The model under review builds one solid part; all positions refer to its coordinate system, in mm. Coordinates: 2 decimals unless noted, no trailing zeros. Loops run counter-clockwise (first coordinate to the right, second up) from the corner with the lowest first, then second, coordinate; pieces in that order, holes last. Notation, with made-up numbers: M 55,-17.5 L 69,-17.5 A4 ccw 69,-11.5 Z; hole C 86,-9.75 d11. An arc over 180 degrees is marked long. Use one line per item in the form item = value.
```python
from build123d import *

# Parameters (mm, degrees)
SKETCH1_R           = 1.524
SKETCH1_W           = 3.175
SKETCH1_H           = 3.175
BOSS_EXTRUDE1_DEPTH = 3.175


with BuildPart() as part:
    # Sketch1 → Boss-Extrude1 (new body)
    with BuildSketch(Plane(origin=(0, 0, 0), x_dir=(0, 0, -1), z_dir=(1, 0, 0))):
        with BuildLine():
            Line((-6.35, -285.75), (6.35, -285.75))
            Line((6.35, -285.75), (10.159096581, -0.135486743))
            ThreePointArc((10.159096581, -0.135486743), (0, 10.16), (-10.159096581, -0.135486743))
            Line((-10.159096581, -0.135486743), (-6.35, -285.75))
        make_face()
        Circle(SKETCH1_R, mode=Mode.SUBTRACT)
        with Locations((0, -10.668)):
            Circle(SKETCH1_R, mode=Mode.SUBTRACT)
        with Locations((0, -5.334)):
            Rectangle(SKETCH1_W, SKETCH1_H, mode=Mode.SUBTRACT)
    extrude(amount=BOSS_EXTRUDE1_DEPTH)


solid = part.part
```
1. Add section C-C (y = -44). State the section outline as (x, z) points (3 decimals).
Response values:
outline = M 0,-9.574 L 3.175,-9.574 L 3.175,9.574 L 0,9.574 Z
2. Add section A-A (x = 2.6). State the section outline as (y, z) points, then the cut area to 3 significant figures.
Response values:
outline = M -285.75,-6.35 L -0.14,-10.16 A10.16 ccw long -0.14,10.16 L -285.75,6.35 Z; hole C -10.67,0 d3.05; hole M -6.92,-1.59 L -3.75,-1.59 L -3.75,1.59 L -6.92,1.59 Z; hole C 0,0 d3.05
area = 4,860 mm^2
3. Insertion check: P1, Ø1.8, axis at y = -10.668, z = 0, coming from the -X side; P2, Ø1.6, axis at x = 2.5, y = -6, coming from the -Z side; P3, Ø5, axis at y = 0, z = 0, coming from the +X side (3 decimals). Each pin has a flat end and moves straight along its axis. Give the tip position at first contact, or say it passes through.
Response values:
P1 = through
P2 = -10.09
P3 = 3.175
4. Add section B-B (y = -139). State the section outline as (x, z) points (3 decimals), then the cut area to 3 significant figures.
Response values:
outline = M 0,-8.307 L 3.175,-8.307 L 3.175,8.307 L 0,8.307 Z
area = 52.8 mm^2
5. Wall thickness on line 1 along Y through (x, z) = (0.3, 0.5); line 2 along Y through (x, z) = (1.85, 0.75); line 3 along Z through (x, y) = (0.6, -44.5): over which ranges is each line inside the solid? List them lowest first. Write a range as from..to.
Response values:
line_1 = -285.75..-12.11, -9.23..-6.92, -3.75..-1.44, 1.44..10.15
line_2 = -285.75..-11.99, -9.34..-6.92, -3.75..-1.33, 1.33..10.13
line_3 = -9.57..9.57
